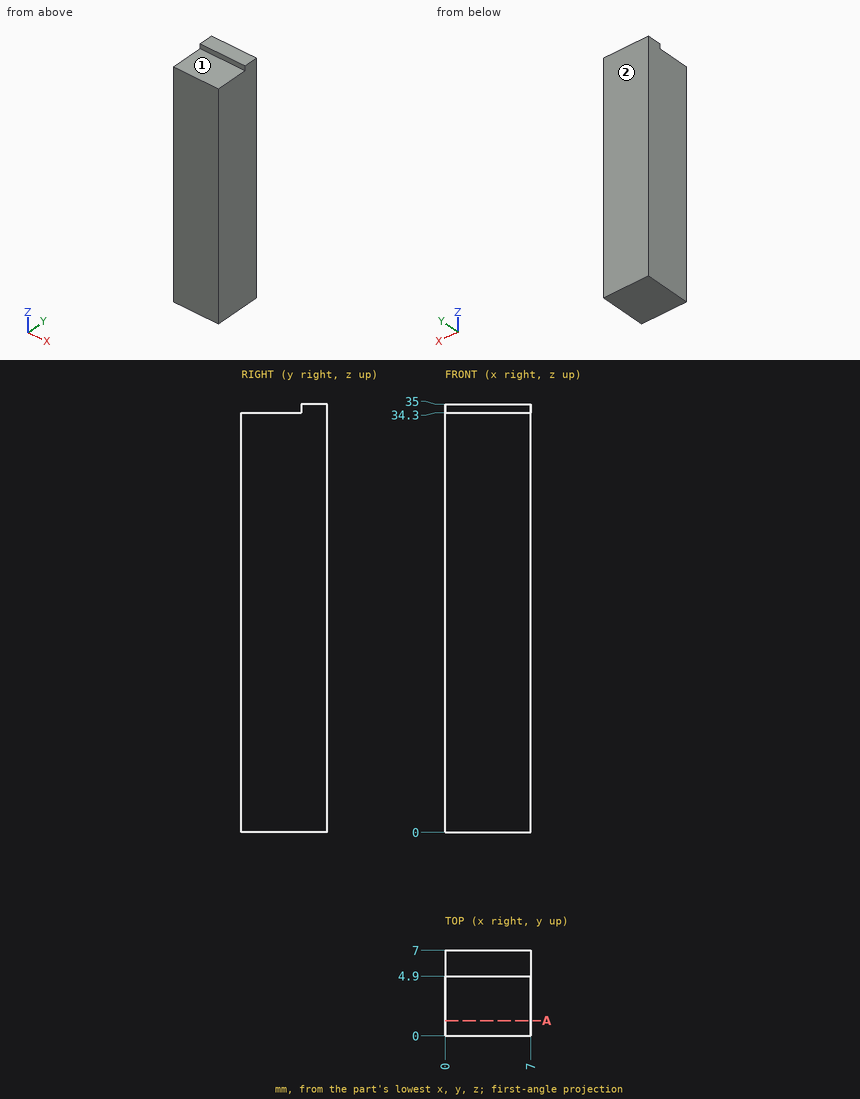
The figure shows three views and two pictorial views of one solid part (mm, origin at its lowest corner). Answer the questions. A direction names the side the tool comes from. Round coordinates to 2 decimals unless told otherwise and drop trailing zeros. Write each loop counter-clockwise with the first axis right and the second up, starting at its lowest first coordinate (ties: lowest second). Pieces come first, ordered by that corner, then holes. Notation, with made-up numbers: M 70.25,78 L 102.25,78 A3 cw 102.25,82 Z; hole C 86,76.5 d4. An arc over 180 degrees is marked long. Write each question's results on one line, items separated by ' | '. Start each with the question number.
(1) The part is cut by section A-A, the plane y = 1.25. Write down the section's boundary in (x, z).
(2) This flat-tipped pin is pushed along its axis until it touches: P1, Ø3, axis at x = 1, y = 1.5, coming from the +Z side. Where does it stop, or does it pass through?
(3) For the marked faces 1 and 2, determine the directions among +Z, -Z, +X, -X, +Y, -Y from which every point of the face is accessible in a straight line to the end or side of a thin tool.
(4) Find the intervals of material crossed by line 1 (Z direction, x = 0.75, y = 2.25), in increasing order.
Worked answers:
1) outline: M 0,0 L 7,0 L 7,34.3 L 0,34.3 Z
2) P1: stops at z = 34.3
3) face 1: +Z, +X, -X, -Y | face 2: +Z, -Z, +X, -X, +Y
4) line 1: z = 0 to 34.3
